The listing builds one solid part. Answer for the finished solid, in the listing's coordinates (mm). Face numbers are marked on the shaded views. A direction names the side the tool comes from. Round coordinates to 2 decimals unless told otherwise and drop trailing zeros. Write each loop counter-clockwise with the first axis right and the second up, starting at its lowest first coordinate (ties: lowest second). Pieces come first, ordered by that corner, then holes.
Item 1: Each of these flat-tipped pins is pushed along its axis until it touches: pin 1 (1.5 mm diameter, centred on y = 1.5, z = 2, fed in from +X); pin 2 (2.5 mm diameter, centred on y = -20.5, z = 2, fed in from -X); pin 3 (3 mm diameter, centred on y = -20.5, z = 4.5, fed in from +X). Where does it stop, or does it pass through?
Item 2: Find the intervals of material crossed by probe 1 along Y at (x, z) = (23.5, 1.15); probe 2 along X at (y, z) = (-21.5, 3.15); probe 3 along X at (y, z) = (-16.5, 2.25), in increasing order.
Item 3: Find section D-D on x = 5.5. Give the vertices of the cut face in (y, z), then the cut area to 3 significant figures.
Item 4: A tool of negligible diameter and unlimited length cuts with its end or side. For the marked faces 1, 2, 3, 4 and 5, from which of +Z, -Z, +X, -X, +Y, -Y can it reach the whole face along a straight path? Write none if from no direction.
Item 5: Find section C-C on x = 39. Give the vertices of the cut face in (y, z), then the cut area to 3 significant figures.
Item 6: For a pull along Y with two mould halves and no side action, classify the marked faces 6, 7 and 8 as +Y half, -Y half, draft (parallel to the pull), parting line (faces both ways), or undercut.
Item 7: Find section A-A on y = -22. Give the vertices of the cut face in (x, z), then the cut area to 3 significant figures.
Item 8: Find section B-B on z = 2.85. Give the vertices of the cut face in (x, y), then the cut area to 3 significant figures.
```python
from build123d import *

# Parameters (mm, degrees)
SKETCH1_W           = 30
SKETCH1_H           = 5
SKETCH1_W_2         = 50
SKETCH1_H_2         = 15
SKETCH1_W_3         = 40
BOSS_EXTRUDE1_DEPTH = 5


with BuildPart() as part:
    # Sketch1 → Boss-Extrude1 (new body)
    # profile 1 of 3: a face of its own
    with BuildSketch(Plane.XY):
        with Locations((25, 2.5)):
            Rectangle(SKETCH1_W, SKETCH1_H)
    # profile 2 of 3: a face of its own
    with BuildSketch(Plane.XY):
        with Locations((25, -7.5)):
            Rectangle(SKETCH1_W_2, SKETCH1_H_2)
    # profile 3 of 3: a face of its own
    with BuildSketch(Plane.XY):
        with Locations((25, -22.5)):
            Rectangle(SKETCH1_W_3, SKETCH1_H_2)
        with Locations((25, -22.5)):
            Rectangle(SKETCH1_W, SKETCH1_H, mode=Mode.SUBTRACT)
    extrude(amount=BOSS_EXTRUDE1_DEPTH)


solid = part.part
```
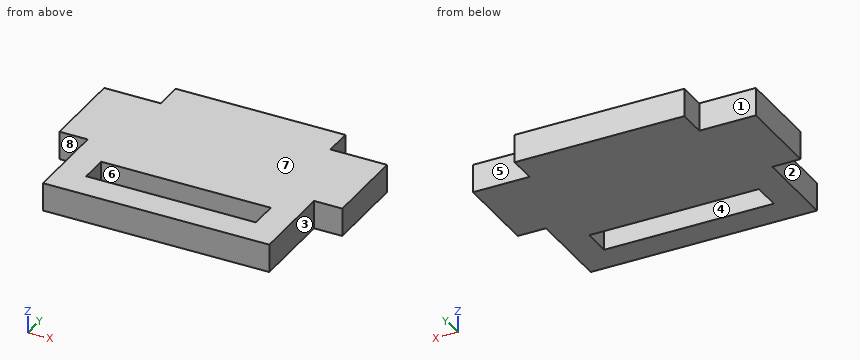
Check values:
1. pin 1: stops at x = 40
1. pin 2: stops at x = 5
1. pin 3: stops at x = 45
2. probe 1: y = -30 to -25, -20 to 5
2. probe 2: x = 5 to 10, 40 to 45
2. probe 3: x = 5 to 45
3. outline: (-30, 0) - (0, 0) - (0, 5) - (-30, 5) - close
3. area: 150 mm2
4. face 1: +Z, -Z, -X, +Y
4. face 2: +Z, -Z, -X, -Y
4. face 3: +Z, -Z, +X, -Y
4. face 4: +Z, -Z
4. face 5: +Z, -Z, +X, +Y
5. outline: (-30, 0) - (-25, 0) - (-25, 5) - (-30, 5) - close; (-20, 0) - (5, 0) - (5, 5) - (-20, 5) - close
5. area: 150 mm2
6. face 6: undercut
6. face 7: draft
6. face 8: -Y half
7. outline: (5, 0) - (10, 0) - (10, 5) - (5, 5) - close; (40, 0) - (45, 0) - (45, 5) - (40, 5) - close
7. area: 50.0 mm2
8. outline: (0, -15) - (5, -15) - (5, -30) - (45, -30) - (45, -15) - (50, -15) - (50, 0) - (40, 0) - (40, 5) - (10, 5) - (10, 0) - (0, 0) - close; hole (10, -25) - (40, -25) - (40, -20) - (10, -20) - close
8. area: 1,350 mm2
